Work out the finished part from the listing and answer in its coordinate system (mm). A direction names the side the tool comes from. Round coordinates to 2 decimals unless told otherwise and drop trailing zeros. Order: outer loops, then holes, each group sorted by start corner. A loop starts at its lowest first (then second) coordinate and runs counter-clockwise, first axis right, second up.
Autodesk Inventor part; units mm, degrees
ref_plane "YZ Plane" through (0, 0, 0) normal (1, 0, 0) x (0, 1, 0)
ref_plane "XZ Plane" through (0, 0, 0) normal (0, 1, 0) x (-1, 0, 0)
ref_plane "XY Plane" through (0, 0, 0) normal (0, 0, 1) x (1, 0, 0)
sketch "草图1" plane through (0, 0, 0) normal (0, 0, 1) x (1, 0, 0)
  circle A0 centre (0, 0) radius 12.75
  dimension "d0" = 25.5
extrude "拉伸1" add sketch "草图1" against normal blind 5
fillet "圆角1" radius 2 1 edges at (-12.75, 0, 0)
shell "抽壳1" thickness 1.5 removed faces 1 at (4.8553, -3.9738, -5)
properties part number "Buttonx26" material "玻璃"
Item 1: Find section D-D (z = -1.2). Write down the section's boundary in (x, y), plus the area to 3 significant figures.
Item 2: Find section A-A (y = 0). Write down the section's boundary in (x, z).
Item 3: Find section C-C (z = -2.85). Write down the section's boundary in (x, y), plus the area to 3 significant figures.
Item 4: A tool of negligible diameter and unlimited length cuts with its end or side. For faces 1 (the face through (7, -9, -5)), 2 (the face through (5.19, -9.98, -3.48)), from which of +Z, -Z, +X, -X, +Y, -Y can it reach the whole face along a straight path? Write none if from no direction.
Item 5: Given pin 1 (1.5 mm diameter, centred on x = -4, z = -2, fed in from -Y); pin 2 (8 mm diameter, centred on x = -5, y = 5, fed in from -Z); pin 3 (2 mm diameter, centred on x = 4, z = -2.5, fed in from -Y), each flat-ended and moving along its own axis, determine where each tip first touches the part or whether it passes through.
Item 6: Find the intervals of material crossed by line 1 along Y through (x, z) = (0, -3.7); line 2 along Z through (x, y) = (-0.5, 6.75); line 3 along Y through (x, z) = (3, -1.95), in increasing order.
Model answer:
1. outline: circle Ø25.17 at (0, 0)
1. area: 497 mm2
2. outline: (-12.75, -5) - (-11.25, -5) - (-11.25, -2) arc R0.5 cw to (-10.75, -1.5) - (10.75, -1.5) arc R0.5 cw to (11.25, -2) - (11.25, -5) - (12.75, -5) - (12.75, -2) arc R2 ccw to (10.75, 0) - (-10.75, 0) arc R2 ccw to (-12.75, -2) - close
3. outline: circle Ø25.5 at (0, 0); hole circle Ø22.5 at (0, 0)
3. area: 113 mm2
4. face 1: -Z, +X, -X, +Y, -Y
4. face 2: -Z
5. pin 1: stops at y = -12.33
5. pin 2: stops at z = -1.62
5. pin 3: stops at y = -12.39
6. line 1: y = -12.75 to -11.25, 11.25 to 12.75
6. line 2: z = -1.5 to 0
6. line 3: y = -12.39 to -10.84, 10.84 to 12.39
